from build123d import *

# Parameters (mm, degrees)
SKETCH1_W                       = 22.225
SKETCH1_H                       = 22.225
BOSS_EXTRUDE1_DEPTH             = 5
F_4_0MM_DOWEL_HOLE3_D           = 4
F_4_0MM_DOWEL_HOLE3_CSINK_D     = 4.05
F_4_0MM_DOWEL_HOLE3_CSINK_ANGLE = 90
CHAMFER1_SIZE                   = 3


with BuildPart() as part:
    # Sketch1 → Boss-Extrude1 (new body)
    with BuildSketch(Plane(origin=(0, 0, 0), x_dir=(1, 0, 0), z_dir=(0, 1, 0))):
        with Locations((11.1125, 11.1125)):
            Rectangle(SKETCH1_W, SKETCH1_H)
    extrude(amount=BOSS_EXTRUDE1_DEPTH)

    # Ø4.0mm Dowel Hole3 (through all)
    with Locations(Plane(origin=(0, 5, 0), x_dir=(1, 0, 0), z_dir=(0, 1, 0))):
        with Locations((7.5, 16.725), (16.725, 7.5)):
            CounterSinkHole(F_4_0MM_DOWEL_HOLE3_D / 2, F_4_0MM_DOWEL_HOLE3_CSINK_D / 2, counter_sink_angle=F_4_0MM_DOWEL_HOLE3_CSINK_ANGLE)

    # Chamfer1
    chamfer1_edges = [part.edges().sort_by_distance(p)[0] for p in [
        (0, 2.5, -22.225),
        (22.225, 2.5, -22.225),
        (22.225, 2.5, 0),
        (0, 2.5, 0),
    ]]
    chamfer(chamfer1_edges, length=CHAMFER1_SIZE)


solid = part.part
The listing builds one solid part. Answer for the finished solid, in the listing's coordinates (mm). Round coordinates to 2 decimals unless told otherwise and drop trailing zeros. Loops run counter-clockwise (first coordinate to the right, second up) from the corner with the lowest first, then second, coordinate; pieces in that order, holes last. Notation, with made-up numbers: M 28.25,41 L 64.25,41 A30 ccw 64.25,67 Z; hole C 13,12.5 d4. An arc over 180 degrees is marked long. Return JSON: item names as keys, results as strings.
Q1. Find the intervals of material crossed by line 1 along Z through (x, y) = (7.5, 1.95) (3 decimals); line 2 along Z through (x, y) = (16.5, 2.25) (3 decimals); line 3 along X through (y, z) = (4, -7) (1 decimal), in increasing order. Write a range as from..to.
Results list:
{"line 1": "z = -22.225..-18.725, -14.725..0", "line 2": "z = -22.225..-9.487, -5.513..0", "line 3": "x = 0..14.8, 18.7..22.2"}
Q2. The mould has two halves that part along X. Classify faces 1 (the face through (20.7, 2.47, -20.75)), 2 (the face through (1.521, 2.465, -20.746)), 3 (the face through (14.817, 2.453, -8.101)): released by +X, released by -X, zero draft, split by the parting line, or undercut.
Results list:
{"face 1": "released by +X", "face 2": "released by -X", "face 3": "undercut"}
Q3. Find section D-D, the plane x = 20.5. Determine the outline of the cut face in (y, z) (3 decimals), plus the area to 3 significant figures.
Results list:
{"outline": "M 0,-20.95 L 5,-20.95 L 5,-1.275 L 0,-1.275 Z", "area": "98.4 mm2"}
Q4. Find section A-A, the plane x = 7.5. Determine the outline of the cut face in (y, z) (3 decimals), plus the area to 3 significant figures.
Results list:
{"outline": "M 0,-22.225 L 5,-22.225 L 5,-18.75 L 4.975,-18.725 L 0,-18.725 Z; M 0,-14.725 L 4.975,-14.725 L 5,-14.7 L 5,0 L 0,0 Z", "area": "91.1 mm2"}
Q5. Find section C-C, the plane y = 4.65. Determine the outline of the cut face in (x, z) (3 decimals).
Results list:
{"outline": "M 0,-19.225 L 3,-22.225 L 19.225,-22.225 L 22.225,-19.225 L 22.225,-3 L 19.225,0 L 3,0 L 0,-3 Z; hole C 7.5,-16.725 d4; hole C 16.725,-7.5 d4"}
Q6. Find section B-B, the plane z = -7.5. Determine the outline of the cut face in (x, y) (3 decimals).
Results list:
{"outline": "M 0,0 L 14.725,0 L 14.725,4.975 L 14.7,5 L 0,5 Z; M 18.725,0 L 22.225,0 L 22.225,5 L 18.75,5 L 18.725,4.975 Z"}
Q7. This flat-tipped pin is pushed along its axis until it touches: pin 1 Ø1 at (x, z) = (15, -14) entering from -Y. Where does it stop, or does it pass through?
Results list:
{"pin 1": "stops at y = 0"}
